from build123d import *

# Parameters (mm, degrees)
BASPROSKE_W        = 130
BASPROSKE_H        = 69
TOOTHCUT_DEPTH     = 163.548454314
TEETHCUTS_COUNT    = 21
TEETHCUTS_ANGLE    = 342.857142857
BORSKE_R           = 32.5
BORE_DEPTH         = 130.0000508
CUT_EXTRUDE1_DEPTH = 163.509966704


with BuildPart() as part:
    # BasProSke → Base-Revolve (revolve)
    with BuildSketch(Plane(origin=(0, 0, 0), x_dir=(1, 0, 0), z_dir=(0, 1, 0)), mode=Mode.PRIVATE) as base_revolve_sk:
        with Locations((65, 34.5)):
            Rectangle(BASPROSKE_W, BASPROSKE_H)
    revolve(base_revolve_sk.sketch.rotate(Axis((-10, 0, 0), (1, 0, 0)), 180), axis=Axis((-10, 0, 0), (1, 0, 0)))

    # TooCutSke → ToothCut (cut, through all)
    with BuildSketch(Plane(origin=(0, 0, 0), x_dir=(0, 0, -1), z_dir=(1, 0, 0))):
        with BuildLine():
            ThreePointArc((2.93985266, 55.421081434), (0, 55.499), (-2.93985266, 55.421081434))
            ThreePointArc((-2.93985266, 55.421081434), (-4.874938915, 62.364127365), (-8.696301499, 68.475398395))
            ThreePointArc((-8.696301499, 68.475398395), (0, 69.0254), (8.696301499, 68.475398395))
            ThreePointArc((8.696301499, 68.475398395), (4.874938915, 62.364127365), (2.93985266, 55.421081434))
        make_face()
    toothcut = extrude(amount=TOOTHCUT_DEPTH, mode=Mode.SUBTRACT)

    # TeethCuts: ToothCut ×21 about axis
    teethcuts_axis = Axis((-10, 0, 0), (1, 0, 0))
    for i in range(1, TEETHCUTS_COUNT):
        add(toothcut.rotate(teethcuts_axis, i * TEETHCUTS_ANGLE / (TEETHCUTS_COUNT - 1)), mode=Mode.SUBTRACT)

    # BorSke → Bore (cut, symmetric)
    with BuildSketch(Plane(origin=(0, 0, 0), x_dir=(0, 0, -1), z_dir=(1, 0, 0))):
        with Locations(Location((0, 0, 0), (0, 0, 180))):
            Circle(BORSKE_R)
    extrude(amount=BORE_DEPTH, both=True, mode=Mode.SUBTRACT)

    # Sketch1 → Cut-Extrude1 (cut, through all)
    with BuildSketch(Plane.ZY):
        Polygon((16.6951355, 35.206852325), (13.284459239, 23.701754001), (1.779360915, 27.112430262), (5.190037177, 38.617528586), align=None)
    extrude(amount=-CUT_EXTRUDE1_DEPTH, mode=Mode.SUBTRACT)


solid = part.part
CAD build for the part. Positions are in the model's coordinates, mm. A direction names the side the tool comes from. Round coordinates to 2 decimals unless told otherwise and drop trailing zeros. Write each loop counter-clockwise with the first axis right and the second up, starting at its lowest first coordinate (ties: lowest second). Pieces come first, ordered by that corner, then holes. Notation, with made-up numbers: M 50,0.25 L 75,0.25 A28 cw 75,31.25 Z; hole C 32.25,-31.75 d6. An arc over 180 degrees is marked long. Put each result on its own line as item: value. Start each with the question number.
1) Drill centre lines: probe 1 along Y at (x, z) = (59, 0); probe 2 along Z at (x, y) = (12, -39.5); probe 3 along Y at (x, z) = (74.5, -62). Where is each one in solid material? Low to high. Write a range as [from, to].
2) Pin check, flat tips, straight feed: pin 1 Ø1 at (x, z) = (111.5, 13.5) entering from -Y; pin 2 Ø1 at (x, y) = (117, -46) entering from +Z; pin 3 Ø6 at (x, z) = (39, -42.5) entering from +Y. Stop position of each tip, or through.
3) Saw through at B-B, the plane y = 9. Write the cut outline in (x, z).
4) Pull direction Z, two halves, no side cores. Call faces 4 (the cylindrical face through (64.09, 42.77, 45.76)), 5 (the cylindrical face through (64.09, 9.467, -61.723)), 6 (the cylindrical face through (64.09, 18.243, -59.92)): pulls with the +Z half, pulls with the -Z half, needs draft (parallel to the pull), parting line crosses it, or undercut.
5) 3-axis set-ups, long thin cutter, end or side, ignore diameter. For faces 1 (the cylindrical face through (64.09, 58.069, 22.965)), 2 (the cylindrical face through (64.09, -9.146, -61.771)), 3 (the cylindrical face through (64.09, 4.19, 55.34)): which of +Z, -Z, +X, -X, +Y, -Y reach the whole face in a straight line?
6) Saw through at A-A, the plane y = 58. Write the cut outline in (x, z), and give its area (3 significant figures).
Resolved:
1. probe 1: [-69, -32.5], [32.5, 55.5]
1. probe 2: [-54.01, -40.96], [-38.99, 38.99], [40.96, 54.01]
1. probe 3: [-26.95, -20.55], [-9.1, -0.01], [9.62, 18.06]
2. pin 1: y = -60.76
2. pin 2: z = 37.81
2. pin 3: y = 51.61
3. outline: M 0,-60.79 L 130,-60.79 L 130,-31.23 L 0,-31.23 Z; M 0,31.23 L 130,31.23 L 130,60.79 L 0,60.79 Z
4. face 4: pulls with the +Z half
4. face 5: pulls with the -Z half
4. face 6: undercut
5. face 1: +X, -X, +Y
5. face 2: +X, -X
5. face 3: +Z, +X, -X
6. outline: M 0,-31.51 L 130,-31.51 L 130,-22.91 L 0,-22.91 Z; M 0,-13.89 L 130,-13.89 L 130,-3.41 L 0,-3.41 Z; M 0,3.41 L 130,3.41 L 130,13.89 L 0,13.89 Z; M 0,22.91 L 130,22.91 L 130,31.51 L 0,31.51 Z
6. area: 4,960 mm²
